```python
from build123d import *

# Parameters (mm, degrees)
F0_W     = 177.8
F0_H     = 44.45
F1_DEPTH = 31.75
F2_W     = 1.5875
F2_H     = 44.45
F3_DEPTH = 3.175


with BuildPart() as f1:
    # F0 (on Top) → F1 (new body)
    with BuildSketch(Plane.XY):
        with Locations((-88.9, -22.225)):
            Rectangle(F0_W, F0_H)
    extrude(amount=F1_DEPTH)

    # F2 (on face) → F3 (cut)
    with BuildSketch(Plane(origin=(0, 0, 0), x_dir=(1, 0, 0), z_dir=(0, 0, -1))):
        with Locations((-23.01875, 22.225)):
            Rectangle(F2_W, F2_H)
        with Locations((-134.9375, 22.225)):
            Rectangle(F2_W, F2_H)
    extrude(amount=-F3_DEPTH, mode=Mode.SUBTRACT)


solid = f1.part
```
The listing builds one solid part. Answer for the finished solid, in the listing's coordinates (mm). A direction names the side the tool comes from. Give positions to 0.01 mm unless a question says otherwise; leave off trailing zeros. Return JSON: item names as keys, results as strings. Group by question number.
1. Determine the mould class of faces 1 (the flat face through (-22.225, -22, 2)), 2 (the flat face through (0, -23, 16)), 3 (the flat face through (-80, -22, 0)) for opening direction X: pulls with the +X half, pulls with the -X half, needs draft (parallel to the pull), parting line crosses it, or undercut.
2. A straight line is drawn through the part: line 1 (X direction, y = -29, z = 2) (1 decimal). Find the intervals that lie inside material, in ascending order. Write a range as [from, to].
3. Given pin 1 Ø0.8 at (x, y) = (-135, -33) entering from -Z (3 decimals), flat-ended and moving along its own axis, determine where the tip first touches the part or whether it passes through.
4. Which of the six approach directions +Z, -Z, +X, -X, +Y, -Y give full straight-line access (tool end or side, diameter ignored) to faces 4 (the flat face through (-90, 0, 16)), 5 (the flat face through (-135.731, -22, 2))?
Verdict:
{
 "1": {"face 1": "undercut", "face 2": "pulls with the +X half", "face 3": "needs draft"},
 "2": {"line 1": "x = [-177.8, -135.7], [-134.1, -23.8], [-22.2, 0]"},
 "3": {"pin 1": "stops at z = 3.175"},
 "4": {"face 4": "+Z, -Z, +X, -X, +Y", "face 5": "-Z, +Y, -Y"}
}
